Here's the drawing with two shaded views (mm, measured from the low corner). I have some questions. Give positions to 0.01 mm unless a question says otherwise; leave off trailing zeros. Write each loop counter-clockwise with the first axis right and the second up, starting at its lowest first coordinate (ties: lowest second). Pieces come first, ordered by that corner, then holes. Notation, with made-up numbers: (53.5, 33.25) - (66.5, 33.25) arc R8 ccw to (66.5, 39.25) - close; hole circle Ø11 at (87.5, -3). An arc over 180 degrees is marked (long way). Answer as a JSON object with one key per item and string values. Group by question number.
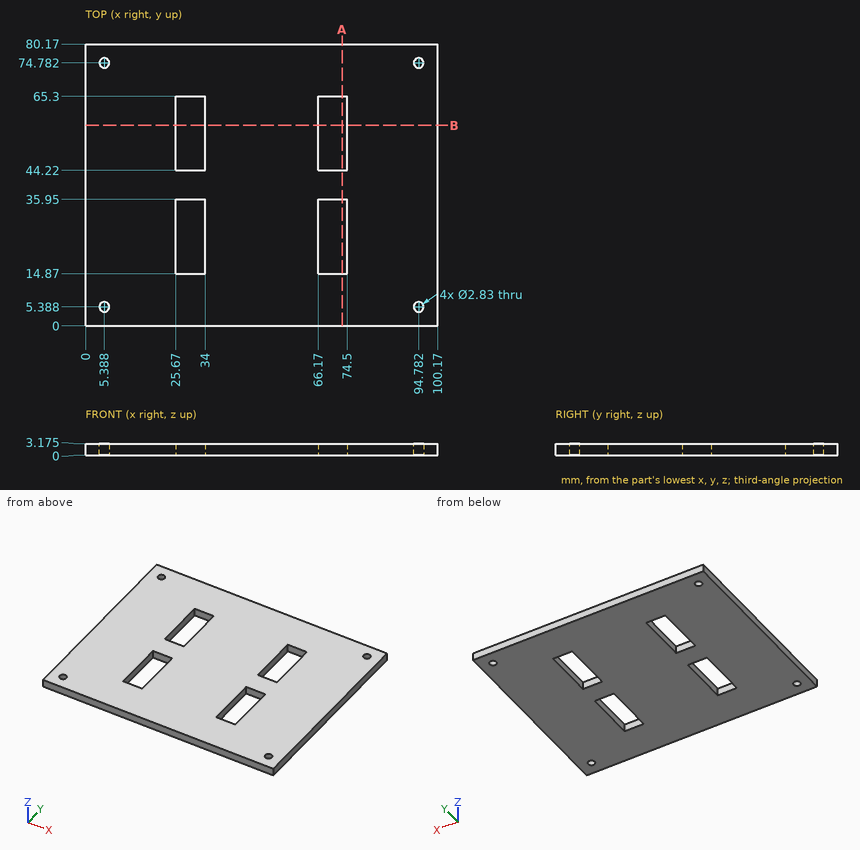
(1) I want a section at B-B, the plane y = 57. Please give me the cut outline in (x, z) (1 decimal), and give its area (3 significant figures).
(2) I need wall thicknesses on L1, parallel to Y at x = 32, z = 0.45; L2, parallel to X at y = 24.5, z = 2.4; L3, parallel to Y at x = 5.5, z = 1.2. Which ranges of each line are inside material? Lowest first, please.
(3) Will these pins go through, and if not, where does the flat tip stop? P1, Ø1, axis at x = 65.5, y = 21.5, coming from the -Z side; P2, Ø1.7, axis at x = 5.39, y = 5.39, coming from the -Z side.
(4) I want a section at A-A, the plane x = 73. State how many separate pieces and enclosed holes the cut face has, and give its area (3 significant figures).
Entries:
{
 "1": {"outline": "(0, 0) - (25.7, 0) - (25.7, 3.2) - (0, 3.2) - close; (34, 0) - (66.2, 0) - (66.2, 3.2) - (34, 3.2) - close; (74.5, 0) - (100.2, 0) - (100.2, 3.2) - (74.5, 3.2) - close", "area": "265 mm^2"},
 "2": {"L1": "0 to 14.87, 35.95 to 44.22, 65.3 to 80.17", "L2": "0 to 25.67, 34 to 66.17, 74.5 to 100.17", "L3": "0 to 3.98, 6.8 to 73.37, 76.19 to 80.17"},
 "3": {"P1": "z = 0", "P2": "through"},
 "4": {"separate pieces": "3", "enclosed holes": "0", "area": "121 mm^2"}
}
